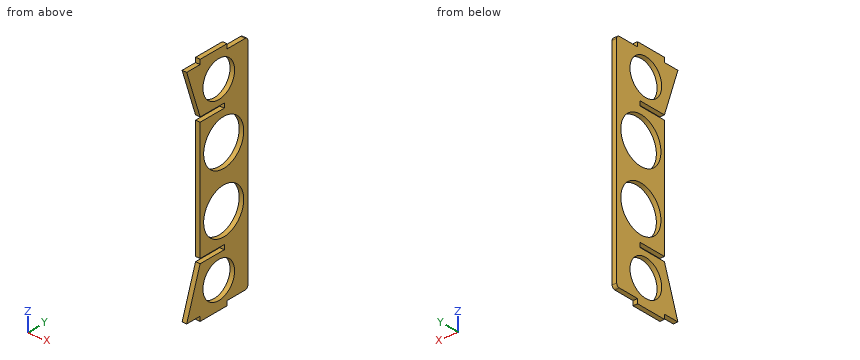
```python
from build123d import *

# Parameters (mm, degrees)
SKETCH1_W           = 144
SKETCH1_H           = 35.5
BOSS_EXTRUDE1_DEPTH = 3
FILLET1_R           = 2
SKETCH2_W           = 3
SKETCH2_H           = 18
CUT_EXTRUDE1_DEPTH  = 3
BOSS_EXTRUDE2_DEPTH = 3
SKETCH4_W           = 3
SKETCH4_H           = 20
BOSS_EXTRUDE3_DEPTH = 3
SKETCH6_R           = 11.782762771
SKETCH6_R_2         = 14.90857156
CUT_EXTRUDE2_DEPTH  = 10


with BuildPart() as part:
    # Sketch1 → Boss-Extrude1 (new body)
    with BuildSketch(Plane(origin=(0, 0, 0), x_dir=(0, 0, -1), z_dir=(1, 0, 0))):
        Rectangle(SKETCH1_W, SKETCH1_H)
    extrude(amount=BOSS_EXTRUDE1_DEPTH)

    # Fillet1
    fillet1_edges = [part.edges().sort_by_distance(p)[0] for p in [
        (1.5, 17.75, 72),
        (1.5, 17.75, -72),
    ]]
    fillet(fillet1_edges, radius=FILLET1_R)

    # Sketch2 → Cut-Extrude1 (cut)
    with BuildSketch(Plane(origin=(3, 0, 0), x_dir=(0, 0, -1), z_dir=(1, 0, 0))):
        with Locations((-40.5, -8.75)):
            Rectangle(SKETCH2_W, SKETCH2_H)
        with Locations((40.5, -8.75)):
            Rectangle(SKETCH2_W, SKETCH2_H)
    extrude(amount=-CUT_EXTRUDE1_DEPTH, mode=Mode.SUBTRACT)

    # Sketch3 → Boss-Extrude2 (add)
    with BuildSketch(Plane(origin=(3, 0, 0), x_dir=(0, 0, -1), z_dir=(1, 0, 0))):
        Polygon((-72, -17.75), (-72, -27.75), (-42, -17.75), align=None)
    boss_extrude2 = extrude(amount=-BOSS_EXTRUDE2_DEPTH)

    # Mirror1: Boss-Extrude2 across plane
    add(boss_extrude2.mirror(Plane.XY))

    # Sketch4 → Boss-Extrude3 (add)
    with BuildSketch(Plane(origin=(3, 0, 0), x_dir=(0, 0, -1), z_dir=(1, 0, 0))):
        with Locations((-73.5, -7.75)):
            Rectangle(SKETCH4_W, SKETCH4_H)
        with Locations((73.5, -7.75)):
            Rectangle(SKETCH4_W, SKETCH4_H)
    extrude(amount=-BOSS_EXTRUDE3_DEPTH)

    # Sketch6 → Cut-Extrude2 (cut)
    with BuildSketch(Plane(origin=(3, 0, 0), x_dir=(0, 0, -1), z_dir=(1, 0, 0))):
        with Locations((-57.483097662, -3.908912232)):
            Circle(SKETCH6_R)
        with Locations((-19.582154149, -0.233669225)):
            Circle(SKETCH6_R_2)
        with Locations((57.483097662, -3.908912232)):
            Circle(SKETCH6_R)
        with Locations((19.582154149, -0.233669225)):
            Circle(SKETCH6_R_2)
    extrude(amount=-CUT_EXTRUDE2_DEPTH, mode=Mode.SUBTRACT)


solid = part.part
```
Part model, mm, in its own coordinate system. Round coordinates to 2 decimals unless told otherwise and drop trailing zeros. Loops run counter-clockwise (first coordinate to the right, second up) from the corner with the lowest first, then second, coordinate; pieces in that order, holes last. Notation, with made-up numbers: (19, 52) -> (67, 52) arc R19 ccw to (67, 62) -> close; hole circle Ø2 at (26, -8). An arc over 180 degrees is marked (long way). Use a Markdown table: item, result.
1) Drop flat-ended pins along their axis: pin 1 Ø0.9 at (x, z) = (1.5, -73.5) entering from +Y; pin 2 Ø0.9 at (x, z) = (1.5, -2) entering from -Y. Give the stop position or say it passes through.
The answers:
| item | result |
|---|---|
| pin 1 | stops at y = 2.25 |
| pin 2 | stops at y = -17.75 |
2) Cut at A-A, the plane y = -25. List the corners of the cut face in (x, z), and give its area (3 significant figures).
The answers:
| item | result |
|---|---|
| outline | (0, -72) -> (3, -72) -> (3, -63.75) -> (0, -63.75) -> close; (0, 63.75) -> (3, 63.75) -> (3, 72) -> (0, 72) -> close |
| area | 49.5 mm2 |
3) Probe line 1 (Z direction, x = 1.35, y = -16); line 2 (Z direction, x = 0.9, y = 4); line 3 (Z direction, x = 2.2, y = 12). List the from-to ranges inside material, lowest first. Write a range as [from, to].
The answers:
| item | result |
|---|---|
| line 1 | z = [-75, -42], [-39, 39], [42, 75] |
| line 2 | z = [-72, -66.22], [-48.75, -33.88], [-5.29, 5.29], [33.88, 48.75], [66.22, 72] |
| line 3 | z = [-72, -28.1], [-11.06, 11.06], [28.1, 72] |
4) Cut at C-C, the plane y = -11. List the corners of the cut face in (x, z).
The answers:
| item | result |
|---|---|
| outline | (0, -75) -> (3, -75) -> (3, -66.89) -> (0, -66.89) -> close; (0, -48.07) -> (3, -48.07) -> (3, -42) -> (0, -42) -> close; (0, -39) -> (3, -39) -> (3, -29.89) -> (0, -29.89) -> close; (0, -9.27) -> (3, -9.27) -> (3, 9.27) -> (0, 9.27) -> close; (0, 29.89) -> (3, 29.89) -> (3, 39) -> (0, 39) -> close; (0, 42) -> (3, 42) -> (3, 48.07) -> (0, 48.07) -> close; (0, 66.89) -> (3, 66.89) -> (3, 75) -> (0, 75) -> close |
5) Cut at B-B, the plane z = 52. List the corners of the cut face in (x, y).
The answers:
| item | result |
|---|---|
| outline | (0, -21.08) -> (3, -21.08) -> (3, -14.34) -> (0, -14.34) -> close; (0, 6.52) -> (3, 6.52) -> (3, 17.75) -> (0, 17.75) -> close |
6) Cut at D-D, the plane x = 2.4. List the corners of the cut face in (y, z), and give its area (3 significant figures).
The answers:
| item | result |
|---|---|
| outline | (-27.75, -72) -> (-17.75, -72) -> (-17.75, -75) -> (2.25, -75) -> (2.25, -72) -> (15.75, -72) arc R2 ccw to (17.75, -70) -> (17.75, 70) arc R2 ccw to (15.75, 72) -> (2.25, 72) -> (2.25, 75) -> (-17.75, 75) -> (-17.75, 72) -> (-27.75, 72) -> (-17.75, 42) -> (0.25, 42) -> (0.25, 39) -> (-17.75, 39) -> (-17.75, -39) -> (0.25, -39) -> (0.25, -42) -> (-17.75, -42) -> close; hole circle Ø23.57 at (-3.91, -57.48); hole circle Ø23.57 at (-3.91, 57.48); hole circle Ø29.82 at (-0.23, -19.58); hole circle Ø29.82 at (-0.23, 19.58) |
| area | 3,150 mm2 |
